from build123d import *

# Parameters (mm, degrees)
F0_R          = 55.495
F1_DEPTH      = 61.11
F2_R          = 42.045
F3_DEPTH      = 1.52
F5_DEPTH      = 30.23
F5_DEPTH_BACK = 92.79
F6_R          = 37.5
F7_DEPTH      = 10.6
F8_R          = 28.5
F9_DEPTH      = 21
F10_R         = 1.7272
F11_DEPTH     = 6.35
F12_W         = 10
F12_H         = 50
F13_DEPTH     = 40
F14_R         = 3
F15_DEPTH     = 10


with BuildPart() as f1:
    # F0 (on Front) → F1 (new body)
    with BuildSketch(Plane.XZ):
        with Locations((20.227775, 17.58517)):
            Circle(F0_R)
    extrude(amount=F1_DEPTH)

    # F2 (on face) → F3 (join)
    with BuildSketch(Plane.XZ.offset(61.11)):
        with Locations((20.227775, 17.58517)):
            Circle(F2_R)
    extrude(amount=F3_DEPTH)

    # F4 (on face) → F5 (join, two sides)
    with BuildSketch(Plane.XZ.offset(62.63)) as f5_sk:
        with BuildLine():
            Line((22.004346, 23.67117), (18.451204, 23.67117))
            ThreePointArc((18.451204, 23.67117), (20.227775, 11.24517), (22.004346, 23.67117))
        make_face()
    extrude(amount=F5_DEPTH)
    extrude(f5_sk.sketch, amount=-F5_DEPTH_BACK)

    # F6 (on face) → F7 (join)
    with BuildSketch(Plane(origin=(0, 0, 0), x_dir=(-1, 0, 0), z_dir=(0, 1, 0))):
        with Locations((-20.227775, 17.58517)):
            Circle(F6_R)
    extrude(amount=F7_DEPTH)

    # F8 (on face) → F9 (join)
    with BuildSketch(Plane(origin=(0, 10.6, 0), x_dir=(-1, 0, 0), z_dir=(0, 1, 0))):
        with Locations((-20.227775, 17.58517)):
            Circle(F8_R)
    extrude(amount=F9_DEPTH)

    # F10 (on face) → F11 (cut)
    with BuildSketch(Plane.XZ.offset(61.11)):
        with Locations((57.043102, 45.876097)):
            Circle(F10_R)
        with Locations((-8.063152, 54.400497)):
            Circle(F10_R)
        with Locations((-16.587552, -10.705758)):
            Circle(F10_R)
        with Locations((48.518702, -19.230158)):
            Circle(F10_R)
    extrude(amount=-F11_DEPTH, mode=Mode.SUBTRACT)

    # F12 (on face) → F13 (join)
    with BuildSketch(Plane(origin=(0, 31.6, 0), x_dir=(-1, 0, 0), z_dir=(0, 1, 0))):
        with Locations((-16.93944, 41.850986)):
            Rectangle(F12_W, F12_H)
    extrude(amount=-F13_DEPTH)

    # F14 (on face) → F15 (cut)
    with BuildSketch(Plane.XZ.offset(92.86)):
        with Locations((20.227775, 17.58517)):
            Circle(F14_R)
    extrude(amount=-F15_DEPTH, mode=Mode.SUBTRACT)


solid = f1.part
Geometry: final body of the model. Coordinates: model frame, mm. A direction names the side the tool comes from. Coordinates: 2 decimals unless noted, no trailing zeros. Order: outer loops, then holes, each group sorted by start corner. A loop starts at its lowest first (then second) coordinate and runs counter-clockwise, first axis right, second up. Notation, with made-up numbers: M -33,74 L 25,74 A18 ccw 25,81 Z; hole C 8.25,36 d10. An arc over 180 degrees is marked long. One line per question, with ' | ' between items. Start each with the question number.
Item 1: Ray query, probe 1 along Y at (x, z) = (55, 20); probe 2 along Y at (x, z) = (12, 17); probe 3 along Z at (x, y) = (-15.5, -58). Return the intervals inside material, ascending. Write a range as [from, to].
Item 2: Cut plane B-B, the plane x = 45. Return the cut outline in (y, z), then the cut area to 3 significant figures.
Item 3: Set-up query: faces 1 (the flat face through (20, -78, 23.671)), 2 (the flat face through (21.939, 20, 56)), 3 (the cylindrical face through (-6.416, -57.979, 54.919)). Return all of +Z, -Z, +X, -X, +Y, -Y with unobstructed straight access to the full face (end or side cutting, diameter ignored); none if empty.
Item 4: Cut plane A-A, the plane z = 26. Return the cut outline in (x, y).
Item 5: Pin query (flat end, axial travel): pin 1 Ø6 at (y, z) = (-26.5, 12) entering from +X; pin 2 Ø4 at (x, y) = (19, -10) entering from -Z; pin 3 Ø3 at (x, z) = (-8.06, 54.4) entering from +Y. Return the tip coordinate at first contact, or that it passes through.
Item 6: Draft query along Z for faces 4 (the flat face through (11.939, 20, 56)), 5 (the cylindrical face through (25.115, 5.226, -19.595)), 6 (the flat face through (20, -82.86, 18)), 7 (the flat face through (17, 16, 66.851)). Return one class per face: released by +Z, released by -Z, zero draft, split by the parting line, or undercut.
Item 7: Cut plane D-D, the plane y = -5.5. Return the cut outline in (x, z) (3 decimals).
Item 8: Cut plane C-C, the plane y = 17. Return the cut outline in (x, z), then the cut area to 3 significant figures.
A:
1) probe 1: y = [-62.63, 10.6] | probe 2: y = [-62.63, 31.6] | probe 3: z = [-24.88, -12.05], [-9.36, 60.05]
2) outline: M -62.63,-16.39 L -61.11,-16.39 L -61.11,-32.07 L 0,-32.07 L 0,-10.57 L 10.6,-10.57 L 10.6,3.49 L 31.6,3.49 L 31.6,31.68 L 10.6,31.68 L 10.6,45.74 L 0,45.74 L 0,67.24 L -61.11,67.24 L -61.11,51.56 L -62.63,51.56 Z | area: 7,360 mm2
3) face 1: +Z, +X, -X, -Y | face 2: +Z, +X, +Y | face 3: -Y
4) outline: M -34.63,-61.11 L -20.97,-61.11 L -20.97,-62.63 L 61.42,-62.63 L 61.42,-61.11 L 75.08,-61.11 L 75.08,0 L 56.77,0 L 56.77,10.6 L 47.46,10.6 L 47.46,31.6 L -7,31.6 L -7,10.6 L -16.32,10.6 L -16.32,0 L -34.63,0 Z
5) pin 1: stops at x = 75.66 | pin 2: stops at z = -37.91 | pin 3: stops at y = 0
6) face 4: zero draft | face 5: split by the parting line | face 6: undercut | face 7: released by +Z
7) outline: C 20.228,17.585 d110.99
8) outline: M 11.94,44.85 A28.5 ccw long 21.94,46.03 L 21.94,66.85 L 11.94,66.85 Z | area: 2,760 mm2
